Can you work these out from the model? Positions are in its coordinate system, mm. Give positions to 0.01 mm unless a question says otherwise; leave off trailing zeros. Loops run counter-clockwise (first coordinate to the right, second up) from the corner with the lowest first, then second, coordinate; pieces in that order, holes last. Notation, with made-up numbers: M 28,-20.75 L 55,-20.75 A22 ccw 55,-13.75 Z; hole C 66,64.5 d5. An arc over 180 degrees is marked long. Put each result on its own line as item: value. Start each with the question number.
1) Imagine slicing it at A-A (x = 0). Write out the boundary of the cut face in (y, z).
2) Please list where these lines run through material, in increasing order: line 1 along Z through (x, y) = (0, 0.65); line 2 along Z through (x, y) = (-1.3, 1.65); line 3 along X through (y, z) = (0.45, -16). Write a range as from..to.
3) Imagine slicing it at B-B (y = 0.7). Write out the boundary of the cut face in (x, z), then the cut area to 3 significant figures.
4) For P1, Ø3, axis at x = 2.5, z = 11, coming from the -Y side; P2, Ø3, axis at x = 0, z = 16, coming from the +Y side, each with a flat end and sliding along its axis, tell me the tip position at first contact or that it passes through.
from build123d import *

# Parameters (mm, degrees)
SKETCH1_R           = 1.25
BOSS_EXTRUDE1_DEPTH = 2
SKETCH2_R           = 2
CUT_EXTRUDE1_DEPTH  = 1
FILLET1_R           = 0.5


with BuildPart() as part:
    # Sketch1 → Boss-Extrude1 (new body)
    with BuildSketch(Plane(origin=(0, 0, 0), x_dir=(1, 0, 0), z_dir=(0, 1, 0))):
        with BuildLine():
            Line((-3, -16), (-3, 16))
            ThreePointArc((-3, 16), (0, 19), (3, 16))
            Line((3, 16), (3, -16))
            ThreePointArc((3, -16), (0, -19), (-3, -16))
        make_face()
        with Locations(Location((0, 16, 0), (0, 0, 270))):
            Circle(SKETCH1_R, mode=Mode.SUBTRACT)
        with Locations(Location((0, -16, 0), (0, 0, 270))):
            Circle(SKETCH1_R, mode=Mode.SUBTRACT)
    extrude(amount=BOSS_EXTRUDE1_DEPTH)

    # Sketch2 → Cut-Extrude1 (cut)
    with BuildSketch(Plane(origin=(0, 2, 0), x_dir=(1, 0, 0), z_dir=(0, 1, 0))):
        with Locations(Location((0, -16, 0), (0, 0, 270))):
            Circle(SKETCH2_R)
        with Locations(Location((0, 16, 0), (0, 0, 90))):
            Circle(SKETCH2_R)
    extrude(amount=-CUT_EXTRUDE1_DEPTH, mode=Mode.SUBTRACT)

    # Fillet1
    fillet1_edges = [part.edges().sort_by_distance(p)[0] for p in [
        (0, 2, -19),
        (-3, 2, 0),
        (0, 1, 14),
        (0, 1, -14),
        (0, 2, 19),
        (3, 2, 0),
    ]]
    fillet(fillet1_edges, radius=FILLET1_R)


solid = part.part
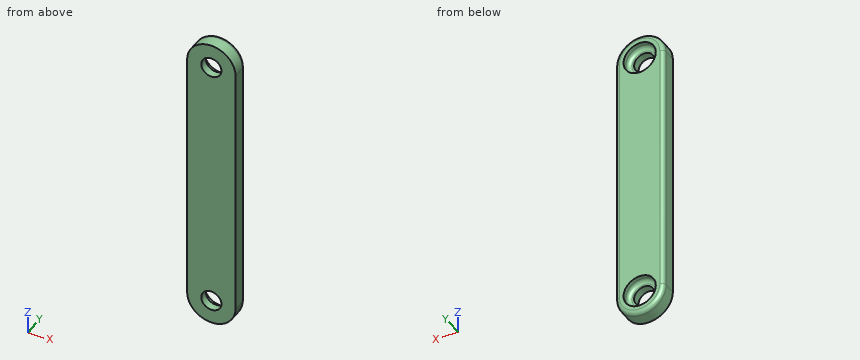
Recorded:
1. outline: M 0,-19 L 1.5,-19 A0.5 ccw 2,-18.5 L 2,-18 L 1.5,-18 A0.5 cw 1,-17.5 L 1,-17.25 L 0,-17.25 Z; M 0,-14.75 L 1,-14.75 L 1,-14.5 A0.5 cw 1.5,-14 L 2,-14 L 2,14 L 1.5,14 A0.5 cw 1,14.5 L 1,14.75 L 0,14.75 Z; M 0,17.25 L 1,17.25 L 1,17.5 A0.5 cw 1.5,18 L 2,18 L 2,18.5 A0.5 ccw 1.5,19 L 0,19 Z
2. line 1: -19..-17.25, -14.75..14.75, 17.25..19
2. line 2: -18.68..-17.52, -14.48..14.48, 17.52..18.68
2. line 3: -3..-1.25, 1.25..3
3. outline: M -3,-16 A3 ccw 3,-16 L 3,16 A3 ccw -3,16 Z; hole C 0,-16 d2.5; hole C 0,16 d2.5
3. area: 210 mm²
4. P1: y = 0
4. P2: y = 1
